from build123d import *

# Parameters (mm, degrees)
ESQUISSE1_R             = 7.75
ESQUISSE1_R_2           = 41.25
ESQUISSE1_R_3           = 6.75
ESQUISSE1_W             = 300
ESQUISSE1_H             = 120
BOSS_EXTRU_1_DEPTH      = 10
CHANFREIN1_SIZE         = 100
ESQUISSE2_W             = 100
ESQUISSE2_H             = 100
ENL_V_MAT_EXTRU_1_DEPTH = 644.544870231
CONG_1_R                = 20
ESQUISSE3_W             = 1497.809837023
ESQUISSE3_H             = 1280.051047864
ENL_V_MAT_EXTRU_2_DEPTH = 644.544870231


with BuildPart() as part:
    # Esquisse1 → Boss.-Extru.1 (new body)
    with BuildSketch(Plane(origin=(0, 0, 0), x_dir=(1, 0, 0), z_dir=(0, 1, 0))):
        Polygon((455, -188.46717088), (455, 188.46717088), (455, 455), (188.46717088, 455), (-188.46717088, 455), (-455, 455), (-455, 188.46717088), (-455, -188.46717088), (-305, -455), (-188.46717088, -455), (188.46717088, -455), (305, -455), align=None)
        with Locations(Location((-255, 0, 0), (0, 0, 270))):
            Circle(ESQUISSE1_R, mode=Mode.SUBTRACT)
        with Locations(Location((-242.519411655, 78.799333566, 0), (0, 0, 270))):
            Circle(ESQUISSE1_R, mode=Mode.SUBTRACT)
        with Locations(Location((-206.299333566, 149.885239335, 0), (0, 0, 270))):
            Circle(ESQUISSE1_R, mode=Mode.SUBTRACT)
        with Locations(Location((-149.885239335, 206.299333566, 0), (0, 0, 270))):
            Circle(ESQUISSE1_R, mode=Mode.SUBTRACT)
        with Locations(Location((-78.799333566, 242.519411655, 0), (0, 0, 270))):
            Circle(ESQUISSE1_R, mode=Mode.SUBTRACT)
        with Locations(Location((0, 255, 0), (0, 0, 270))):
            Circle(ESQUISSE1_R, mode=Mode.SUBTRACT)
        with Locations(Location((78.799333566, 242.519411655, 0), (0, 0, 270))):
            Circle(ESQUISSE1_R, mode=Mode.SUBTRACT)
        with Locations(Location((149.885239335, 206.299333566, 0), (0, 0, 270))):
            Circle(ESQUISSE1_R, mode=Mode.SUBTRACT)
        with Locations(Location((206.299333566, 149.885239335, 0), (0, 0, 270))):
            Circle(ESQUISSE1_R, mode=Mode.SUBTRACT)
        with Locations(Location((242.519411655, 78.799333566, 0), (0, 0, 270))):
            Circle(ESQUISSE1_R, mode=Mode.SUBTRACT)
        with Locations(Location((255, 0, 0), (0, 0, 270))):
            Circle(ESQUISSE1_R, mode=Mode.SUBTRACT)
        with Locations(Location((242.519411655, -78.799333566, 0), (0, 0, 270))):
            Circle(ESQUISSE1_R, mode=Mode.SUBTRACT)
        with Locations(Location((206.299333566, -149.885239335, 0), (0, 0, 270))):
            Circle(ESQUISSE1_R, mode=Mode.SUBTRACT)
        with Locations(Location((149.885239335, -206.299333566, 0), (0, 0, 270))):
            Circle(ESQUISSE1_R, mode=Mode.SUBTRACT)
        with Locations(Location((78.799333566, -242.519411655, 0), (0, 0, 270))):
            Circle(ESQUISSE1_R, mode=Mode.SUBTRACT)
        with Locations(Location((0, -255, 0), (0, 0, 270))):
            Circle(ESQUISSE1_R, mode=Mode.SUBTRACT)
        with Locations(Location((-78.799333566, -242.519411655, 0), (0, 0, 270))):
            Circle(ESQUISSE1_R, mode=Mode.SUBTRACT)
        with Locations(Location((-149.885239335, -206.299333566, 0), (0, 0, 270))):
            Circle(ESQUISSE1_R, mode=Mode.SUBTRACT)
        with Locations(Location((-206.299333566, -149.885239335, 0), (0, 0, 270))):
            Circle(ESQUISSE1_R, mode=Mode.SUBTRACT)
        with Locations(Location((-242.519411655, -78.799333566, 0), (0, 0, 270))):
            Circle(ESQUISSE1_R, mode=Mode.SUBTRACT)
        with Locations(Location((70, 372.479529639, 0), (0, 0, 270))):
            Circle(ESQUISSE1_R_2, mode=Mode.SUBTRACT)
        with Locations(Location((123, 372.479529639, 0), (0, 0, 270))):
            Circle(ESQUISSE1_R_3, mode=Mode.SUBTRACT)
        with Locations(Location((17, 372.479529639, 0), (0, 0, 270))):
            Circle(ESQUISSE1_R_3, mode=Mode.SUBTRACT)
        with Locations(Location((-17, 372.479529639, 0), (0, 0, 90))):
            Circle(ESQUISSE1_R_3, mode=Mode.SUBTRACT)
        with Locations(Location((-123, 372.479529639, 0), (0, 0, 90))):
            Circle(ESQUISSE1_R_3, mode=Mode.SUBTRACT)
        with Locations(Location((-70, 372.479529639, 0), (0, 0, 90))):
            Circle(ESQUISSE1_R_2, mode=Mode.SUBTRACT)
        with Locations(Location((372.479529639, 70, 0), (0, 0, 90))):
            Circle(ESQUISSE1_R_2, mode=Mode.SUBTRACT)
        with Locations(Location((372.479529639, 17, 0), (0, 0, 90))):
            Circle(ESQUISSE1_R_3, mode=Mode.SUBTRACT)
        with Locations(Location((372.479529639, 123, 0), (0, 0, 90))):
            Circle(ESQUISSE1_R_3, mode=Mode.SUBTRACT)
        with Locations(Location((372.479529639, -70, 0), (0, 0, 270))):
            Circle(ESQUISSE1_R_2, mode=Mode.SUBTRACT)
        with Locations(Location((372.479529639, -123, 0), (0, 0, 270))):
            Circle(ESQUISSE1_R_3, mode=Mode.SUBTRACT)
        with Locations(Location((372.479529639, -17, 0), (0, 0, 270))):
            Circle(ESQUISSE1_R_3, mode=Mode.SUBTRACT)
        with Locations(Location((70, -372.479529639, 0), (0, 0, 90))):
            Circle(ESQUISSE1_R_2, mode=Mode.SUBTRACT)
        with Locations(Location((17, -372.479529639, 0), (0, 0, 90))):
            Circle(ESQUISSE1_R_3, mode=Mode.SUBTRACT)
        with Locations(Location((123, -372.479529639, 0), (0, 0, 90))):
            Circle(ESQUISSE1_R_3, mode=Mode.SUBTRACT)
        with Locations(Location((-70, -372.479529639, 0), (0, 0, 270))):
            Circle(ESQUISSE1_R_2, mode=Mode.SUBTRACT)
        with Locations(Location((-123, -372.479529639, 0), (0, 0, 270))):
            Circle(ESQUISSE1_R_3, mode=Mode.SUBTRACT)
        with Locations(Location((-17, -372.479529639, 0), (0, 0, 270))):
            Circle(ESQUISSE1_R_3, mode=Mode.SUBTRACT)
        with Locations(Location((-372.479529639, -70, 0), (0, 0, 90))):
            Circle(ESQUISSE1_R_2, mode=Mode.SUBTRACT)
        with Locations(Location((-372.479529639, -17, 0), (0, 0, 90))):
            Circle(ESQUISSE1_R_3, mode=Mode.SUBTRACT)
        with Locations(Location((-372.479529639, -123, 0), (0, 0, 90))):
            Circle(ESQUISSE1_R_3, mode=Mode.SUBTRACT)
        with Locations(Location((-372.479529639, 70, 0), (0, 0, 270))):
            Circle(ESQUISSE1_R_2, mode=Mode.SUBTRACT)
        with Locations(Location((-372.479529639, 123, 0), (0, 0, 270))):
            Circle(ESQUISSE1_R_3, mode=Mode.SUBTRACT)
        with Locations(Location((-372.479529639, 17, 0), (0, 0, 270))):
            Circle(ESQUISSE1_R_3, mode=Mode.SUBTRACT)
        with Locations((0, 100)):
            Rectangle(ESQUISSE1_W, ESQUISSE1_H, mode=Mode.SUBTRACT)
    extrude(amount=BOSS_EXTRU_1_DEPTH)

    # Chanfrein1
    chanfrein1_edges = [part.edges().sort_by_distance(p)[0] for p in [
        (-455, 5, -455),
        (455, 5, -455),
    ]]
    chamfer(chanfrein1_edges, length=CHANFREIN1_SIZE)

    # Esquisse2 → Enlèv. mat.-Extru.1 (cut, through all)
    with BuildSketch(Plane(origin=(0, 10, 0), x_dir=(1, 0, 0), z_dir=(0, 1, 0))):
        with Locations((-275, 275)):
            Rectangle(ESQUISSE2_W, ESQUISSE2_H)
        with Locations((275, 275)):
            Rectangle(ESQUISSE2_W, ESQUISSE2_H)
    extrude(amount=-ENL_V_MAT_EXTRU_1_DEPTH, mode=Mode.SUBTRACT)

    # Congé1
    cong_1_edges = [part.edges().sort_by_distance(p)[0] for p in [
        (-150, 5, -160),
        (-150, 5, -40),
        (150, 5, -40),
        (150, 5, -160),
        (-325, 5, -225),
        (-325, 5, -325),
        (-225, 5, -325),
        (-225, 5, -225),
        (225, 5, -325),
        (325, 5, -325),
        (325, 5, -225),
        (225, 5, -225),
    ]]
    fillet(cong_1_edges, radius=CONG_1_R)

    # Esquisse3 → Enlèv. mat.-Extru.2 (cut, through all)
    with BuildSketch(Plane(origin=(0, 10, 0), x_dir=(1, 0, 0), z_dir=(0, 1, 0))):
        with Locations((34.907275201, -41.538880661)):
            Rectangle(ESQUISSE3_W, ESQUISSE3_H)
        Polygon((30, -445), (-30, -445), (-30, -455), (-120, -455), (-120, -445), (-180, -445), (-180, -455), (-270, -455), (-270, -445), (-299.152964676, -445), (-312.431510738, -421.405543677), (-321.146214104, -426.310025835), (-365.286553526, -347.877695539), (-356.57185016, -342.973213381), (-385.998743108, -290.684993183), (-394.713446474, -295.589475341), (-438.853785896, -217.157145045), (-430.13908253, -212.252662887), (-445, -185.846513709), (-445, -112.494324666), (-455, -112.494324666), (-455, -22.494324666), (-445, -22.494324666), (-445, 37.505675334), (-455, 37.505675334), (-455, 127.505675334), (-445, 127.505675334), (-445, 187.505675334), (-455, 187.505675334), (-455, 277.505675334), (-445, 277.505675334), (-445, 350.857864376), (-429.748737342, 366.109127035), (-436.819805153, 373.180194847), (-373.180194847, 436.819805153), (-366.109127035, 429.748737342), (-350.857864376, 445), (-280, 445), (-280, 455), (-190, 455), (-190, 445), (-130, 445), (-130, 455), (-40, 455), (-40, 445), (40, 445), (40, 455), (130, 455), (130, 445), (190, 445), (190, 455), (280, 455), (280, 445), (350.857864376, 445), (366.109127035, 429.748737342), (373.180194847, 436.819805153), (436.819805153, 373.180194847), (429.748737342, 366.109127035), (445, 350.857864376), (445, 277.505675334), (455, 277.505675334), (455, 187.505675334), (445, 187.505675334), (445, 127.505675334), (455, 127.505675334), (455, 37.505675334), (445, 37.505675334), (445, -22.494324666), (455, -22.494324666), (455, -112.494324666), (445, -112.494324666), (445, -185.846513709), (430.13908253, -212.252662887), (438.853785896, -217.157145045), (394.713446474, -295.589475341), (385.998743108, -290.684993183), (356.57185016, -342.973213381), (365.286553526, -347.877695539), (321.146214104, -426.310025835), (312.431510738, -421.405543677), (299.152964676, -445), (270, -445), (270, -455), (180, -455), (180, -445), (120, -445), (120, -455), (30, -455), align=None, mode=Mode.SUBTRACT)
    extrude(amount=-ENL_V_MAT_EXTRU_2_DEPTH, mode=Mode.SUBTRACT)


solid = part.part
Model file for the job. Use its own axes, mm. A direction names the side the tool comes from. Round coordinates to 2 decimals unless told otherwise and drop trailing zeros. Loops run counter-clockwise (first coordinate to the right, second up) from the corner with the lowest first, then second, coordinate; pieces in that order, holes last. Notation, with made-up numbers: (29.25, 35.25) -> (54.25, 35.25) arc R11 cw to (54.25, 46.25) -> close; hole circle Ø11 at (-10, -2.5). An arc over 180 degrees is marked (long way). Answer as CSV lines item,"result". Start each with the question number.
1) Slice it at A-A (x = 57.5). List the corners of the cut face in (y, z), plus the area to 3 significant figures.
2) Mould opens along X. For faces 3 (the face through (405, 5, -405)), 4 (the face through (231.014, 4.93, -319.297)), 5 (the face through (-318.986, 4.93, -230.703)), 6 (the face through (-6, 0, -6)) say: +X half, -X half, draft (parallel to the pull), parting line (faces both ways), or undercut.
3) Pin check, flat tips, straight feed: P1, Ø4, axis at x = 155.5, y = 9, coming from the +Z side; P2, Ø8, axis at x = -372.48, z = 123, coming from the -Y side; P3, Ø3, axis at x = -282.5, y = 3.5, coming from the -Z side; P4, Ø1.5, axis at y = 8.5, z = 221.5, coming from the -X side. Stop position of each tip, or through.
4) Probe line 1 along Z through (x, y) = (-207, 6.5); line 2 along X through (y, z) = (6, -87); line 3 along X through (y, z) = (5, 47). List the from-to ranges inside material, lowest first.
5) Tool access for faces 1 (the face through (-144.297, 5.07, -153.986)), 2 (the face through (342.91, 4.93, 387.64)): list every direction of +Z, -Z, +X, -X, +Y, -Y with a clear straight run to the whole face (end or side of a thin tool).
6) Slice it at B-B (y = 7.5). State how many separate pieces and enclosed holes the cut face has, plus the area to 3 significant figures.
Filled in:
1,outline,"(0, -455) -> (10, -455) -> (10, -411.79) -> (0, -411.79) -> close; (0, -333.17) -> (10, -333.17) -> (10, -160) -> (0, -160) -> close; (0, -40) -> (10, -40) -> (10, 333.17) -> (0, 333.17) -> close; (0, 411.79) -> (10, 411.79) -> (10, 455) -> (0, 455) -> close"
1,area,"6,330 mm2"
2,face 3,"+X half"
2,face 4,"undercut"
2,face 5,"undercut"
2,face 6,"draft"
3,P1,"stops at z = 445"
3,P2,"passes through"
3,P3,"stops at z = -445"
3,P4,"stops at x = -436.83"
4,line 1,"z = -455 to -157.6, -142.17 to 142.17, 157.6 to 455"
4,line 2,"x = -455 to -410.06, -334.9 to -150, 150 to 334.9, 410.06 to 455"
4,line 3,"x = -455 to -406.72, -338.24 to 338.24, 406.72 to 455"
5,face 1,"+Y, -Y"
5,face 2,"+Z, +X, +Y, -Y"
6,separate pieces,"1"
6,enclosed holes,"47"
6,area,"660,000 mm2"
